Here's how the part is built. I have some questions about the finished solid (model axes, mm). A direction names the side the tool comes from. Round coordinates to 2 decimals unless told otherwise and drop trailing zeros. Write each loop counter-clockwise with the first axis right and the second up, starting at its lowest first coordinate (ties: lowest second). Pieces come first, ordered by that corner, then holes. Notation, with made-up numbers: (52, 50) -> (56, 50) arc R5 cw to (56, 54) -> close; hole circle Ø9 at (4.5, -7). An arc over 180 degrees is marked (long way). Put each result on its own line as item: value. Start each with the question number.
1. Suppose I cut it at A-A (z = 0). Please give me the cut outline in (x, y).
2. Suppose I cut it at B-B (x = 0). Please give me the cut outline in (y, z).
3. Suppose I cut it at C-C (y = -7.25). Please give me the cut outline in (x, z).
4. Which directions (+Z, -Z, +X, -X, +Y, -Y) give clear straight access to the entire face, cutting with the end or side of a thin tool? Please do faces 1 (the face through (-5, -2.5, 5)), 2 (the face through (-1, 0, -8)).
5. Suppose I cut it at D-D (z = 33). Please give me the cut outline in (x, y), then the cut area to 3 significant figures.
6. We'd pull the mould along X, two halves only. Please class faces 3 (the face through (7.3, -9.75, -8.3)), 4 (the face through (-3.2, -6.1, 10)), 5 (the face through (23.122, -4.31, -30.156)): +X half, -X half, draft (parallel to the pull), parting line (faces both ways), or undercut.
7. I need wall thicknesses on probe 1 along X at (y, z) = (-3.25, 0); probe 2 along Z at (x, y) = (-16, -7.5); probe 3 along X at (y, z) = (-0.65, 0). Which ranges of each line are inside material? Lowest first, please. Write a range as from..to.
8. For pin 1 (1.5 mm diameter, centred on x = 21.5, y = -4, fed in from +Z); pin 2 (2 mm diameter, centred on x = -17, y = -6, fed in from +Z); pin 3 (5 mm diameter, centred on x = -12, y = -7.5, fed in from -Z), each with a flat end and sliding along its axis, tell me the tip position at first contact or that it passes through.
```python
from build123d import *

# Parameters (mm, degrees)
SKETCH2_R          = 1
CUT_EXTRUDE1_DEPTH = 55.617419382


with BuildPart() as part:
    # Sketch1 → Revolve1 (revolve)
    with BuildSketch(Plane.XY, mode=Mode.PRIVATE) as revolve1_sk:
        Polygon((-6.5, 0), (-38, 0), (-38, -8.5), (-35, -8.5), (-35, -9.75), (-10.5, -9.75), (-10.5, -2.5), (-6.5, -2.5), align=None)
    revolve(revolve1_sk.sketch.rotate(Axis((0, 38.708668819, 0), (0, -1, 0)), 270), axis=Axis((0, 38.708668819, 0), (0, -1, 0)))

    # Sketch2 → Cut-Extrude1 (cut, through all)
    with BuildSketch(Plane.XZ.offset(9.75)):
        with Locations(Location((-33.26875, 0, 0), (0, 0, 270))):
            Circle(SKETCH2_R)
        with Locations(Location((-16.634375, 28.811582652, 0), (0, 0, 270))):
            Circle(SKETCH2_R)
        with Locations(Location((16.634375, 28.811582652, 0), (0, 0, 270))):
            Circle(SKETCH2_R)
        with Locations(Location((33.26875, 0, 0), (0, 0, 270))):
            Circle(SKETCH2_R)
        with Locations(Location((16.634375, -28.811582652, 0), (0, 0, 270))):
            Circle(SKETCH2_R)
        with Locations(Location((-16.634375, -28.811582652, 0), (0, 0, 270))):
            Circle(SKETCH2_R)
    extrude(amount=-CUT_EXTRUDE1_DEPTH, mode=Mode.SUBTRACT)


solid = part.part
```
Verdict:
1. outline: (-38, -8.5) -> (-35, -8.5) -> (-35, -9.75) -> (-34.27, -9.75) -> (-34.27, 0) -> (-38, 0) -> close; (-32.27, -9.75) -> (-10.5, -9.75) -> (-10.5, -2.5) -> (-6.5, -2.5) -> (-6.5, 0) -> (-32.27, 0) -> close; (6.5, -2.5) -> (10.5, -2.5) -> (10.5, -9.75) -> (32.27, -9.75) -> (32.27, 0) -> (6.5, 0) -> close; (34.27, -9.75) -> (35, -9.75) -> (35, -8.5) -> (38, -8.5) -> (38, 0) -> (34.27, 0) -> close
2. outline: (-9.75, -35) -> (-8.5, -35) -> (-8.5, -38) -> (0, -38) -> (0, -6.5) -> (-2.5, -6.5) -> (-2.5, -10.5) -> (-9.75, -10.5) -> close; (-9.75, 10.5) -> (-2.5, 10.5) -> (-2.5, 6.5) -> (0, 6.5) -> (0, 38) -> (-8.5, 38) -> (-8.5, 35) -> (-9.75, 35) -> close
3. outline: circle Ø76 at (0, 0); hole circle Ø2 at (-33.27, 0); hole circle Ø2 at (-16.63, -28.81); hole circle Ø2 at (-16.63, 28.81); hole circle Ø21 at (0, 0); hole circle Ø2 at (16.63, -28.81); hole circle Ø2 at (16.63, 28.81); hole circle Ø2 at (33.27, 0)
4. face 1: -Y
4. face 2: +Z, -Z, +X, -X, +Y
5. outline: (-18.84, -8.5) -> (-11.66, -8.5) -> (-11.66, -9.75) -> (11.66, -9.75) -> (11.66, -8.5) -> (18.84, -8.5) -> (18.84, 0) -> (-18.84, 0) -> close
5. area: 349 mm^2
6. face 3: draft
6. face 4: undercut
6. face 5: parting line
7. probe 1: x = -38..-34.27, -32.27..-10.5, 10.5..32.27, 34.27..38
7. probe 2: z = -34.47..-29.58, -28.04..28.04, 29.58..34.47
7. probe 3: x = -38..-34.27, -32.27..-6.5, 6.5..32.27, 34.27..38
8. pin 1: stops at z = 31.83
8. pin 2: stops at z = 34.47
8. pin 3: stops at z = -36.79
